from build123d import *

# Parameters (mm, degrees)
ENL_V_MAT_EXTRU_1_DEPTH = 1.5


with BuildPart() as part:
    # Esquisse1 → Révolution1 (revolve)
    with BuildSketch(Plane(origin=(0, 0, 0), x_dir=(1, 0, 0), z_dir=(0, 1, 0))):
        Polygon((-1.3, 0), (-1.3, 2.5), (0, 2.5), (0, 1.25), (7.724, 1.25), (8, 0.974), (8, 0), align=None)
    revolve(axis=Axis((8, 0, 0), (-1, 0, 0)))

    # Esquisse2 → Enlèvement de matière-Révolution1 (revolve, cut)
    with BuildSketch(Plane.XY):
        Polygon((-1.3, 0), (-1.3, 0.75055535), (-1.19944465, 0.65), (0.2, 0.65), (0.575277675, 0), align=None)
    revolve(axis=Axis((0.575277675, 0, 0), (-1, 0, 0)), mode=Mode.SUBTRACT)

    # Esquisse3 → Enlèv. mat.-Extru.1 (cut)
    with BuildSketch(Plane(origin=(-1.3, 0, 0), x_dir=(0, 0, -1), z_dir=(1, 0, 0))):
        Polygon((-0.65, 0.375277675), (-0.65, -0.375277675), (0, -0.75055535), (0.65, -0.375277675), (0.65, 0.375277675), (0, 0.75055535), align=None)
    extrude(amount=ENL_V_MAT_EXTRU_1_DEPTH, mode=Mode.SUBTRACT)


solid = part.part
The listing builds one solid part. Answer for the finished solid, in the listing's coordinates (mm). A direction names the side the tool comes from. Give positions to 0.01 mm unless a question says otherwise; leave off trailing zeros. Write each loop counter-clockwise with the first axis right and the second up, starting at its lowest first coordinate (ties: lowest second). Pieces come first, ordered by that corner, then holes. Notation, with made-up numbers: (-9, 29) - (17, 29) arc R28 ccw to (17, 66) - close; hole circle Ø10 at (-22.5, 39). An arc over 180 degrees is marked (long way). Use a Markdown table: item, result.
1. Section A-A on y = -1.65 is taken. Write down the section's boundary in (x, z), plus the area to 3 significant figures.
Values follow:
| item | result |
|---|---|
| outline | (-1.3, -1.88) - (0, -1.88) - (0, 1.88) - (-1.3, 1.88) - close |
| area | 4.88 mm² |
2. Find the intervals of material crossed by probe 1 along X at (y, z) = (-1.6, -0.5); probe 2 along Z at (x, y) = (0.5, 1); probe 3 along Z at (x, y) = (4.25, -1.1), in increasing order. Write a range as from..to.
Values follow:
| item | result |
|---|---|
| probe 1 | x = -1.3..0 |
| probe 2 | z = -0.75..0.75 |
| probe 3 | z = -0.59..0.59 |
3. For a pull along Z with two mould halves and no side action, classify faces 3 (the conical face through (0.515, -0.082, 0.063)), 4 (the cylindrical face through (3.92, 1.22, 0.27)), 5 (the flat face through (8, 0, 0)) as released by +Z, released by -Z, zero draft, split by the parting line, or undercut.
Values follow:
| item | result |
|---|---|
| face 3 | undercut |
| face 4 | split by the parting line |
| face 5 | zero draft |
4. A tool of negligible diameter and unlimited length cuts with its end or side. For faces 1 (the cylindrical face through (-0.64, 2.44, 0.54)), 2 (the flat face through (0, -1, -1)), from which of +Z, -Z, +X, -X, +Y, -Y can it reach the whole face along a straight path? Write none if from no direction.
Values follow:
| item | result |
|---|---|
| face 1 | +X, -X |
| face 2 | +X |
5. Each of these flat-tipped pins is pushed along its axis until it touches: P1, Ø1.5, axis at x = 4, y = 0.5, coming from the +Z side; P2, Ø1, axis at x = 1.5, z = 0, coming from the +Y side; P3, Ø3, axis at x = 2, y = -2, coming from the +Z side. Where does it stop, or does it pass through?
Values follow:
| item | result |
|---|---|
| P1 | stops at z = 1.25 |
| P2 | stops at y = 1.25 |
| P3 | stops at z = 1.15 |
6. Section B-B on z = -1.9 is taken. Write down the section's boundary in (x, y).
Values follow:
| item | result |
|---|---|
| outline | (-1.3, -1.62) - (0, -1.62) - (0, 1.62) - (-1.3, 1.62) - close |
